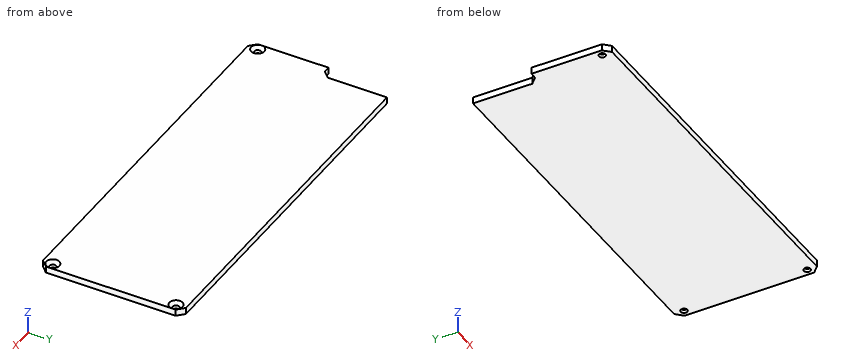
Autodesk Inventor part; units mm, degrees
ref_plane "YZ Plane" through (0, 0, 0) normal (1, 0, 0) x (0, 1, 0)
ref_plane "XZ Plane" through (0, 0, 0) normal (0, 1, 0) x (-1, 0, 0)
ref_plane "XY Plane" through (0, 0, 0) normal (0, 0, 1) x (1, 0, 0)
sketch "Sketch1" plane through (0, 0, 0) normal (1, 0, 0) x (0, 1, 0)
  point P0 (0, 0)
sketch "Sketch2" plane through (0, 0, 0) normal (0, 0, 1) x (1, 0, 0)
  line L0 (-65.94, 18.9) -> (48.46, 18.9)
  line L1 (48.46, 18.9) -> (48.46, -24.5)
  line L2 (48.46, -24.5) -> (-65.94, -24.5)
  line L3 (-65.94, -24.5) -> (-65.94, 18.9)
  point P0 (0, 0)
  dimension "d0" = 43.4
  dimension "d1" = 114.4
extrude "Extrusion1" add sketch "Sketch2" along normal blind 2
chamfer "Chamfer1" distance 2 angle 45 3 edges at (48.46, 18.9, 1) (48.46, -24.5, 1) (-65.94, -24.5, 1)
sketch "Sketch3" plane through (0, 0, 2) normal (0, 0, 1) x (1, 0, 0)
  line L0 (-65.94, 18.9) -> (-61.94, 18.9)
  line L1 (-61.94, 18.9) -> (-61.94, -1.1)
  line L2 (-61.94, -1.1) -> (-65.94, -1.1)
  line L3 (-65.94, -1.1) -> (-65.94, 18.9)
  point P0 (0, 0)
  dimension "d7" = 4
  dimension "d8" = 20
extrude "Extrusion2" cut sketch "Sketch3" against normal blind 2
chamfer "Chamfer2" distance 2 angle 45 1 edges at (-61.94, -1.1, 1)
sketch "Sketch4" plane through (0, 0, 2) normal (0, 0, 1) x (1, 0, 0)
  line L0 (-61.94, 18.9) -> (46.46, 18.9)
  line L1 (-63.94, -24.5) -> (46.46, -24.5)
  line L2 (48.46, -22.5) -> (48.46, 16.9)
  line L3 (-65.94, -22.5) -> (-65.94, -1.1)
  point P0 (0, 0)
  point P1 (-63.94, -21.5)
  point P2 (46.46, -21.5)
  point P3 (46.46, 15.9)
  dimension "d14" = 3
  dimension "d15" = 3
  dimension "d16" = 2
  dimension "d17" = 2
  dimension "d18" = 2
  dimension "d19" = 3
hole "Hole1" at (-63.94, -21.5, 2) at (46.46, -21.5, 2) at (46.46, 15.9, 2) direction (0, 0, -1) diameter 2 depth 8 tip angle 118 countersink diameter 4 countersink angle 90
properties part number "main body cover"
Source: CAD feature listing. Evaluate the final solid. Frame: model axes, mm. Round coordinates to 2 decimals unless told otherwise and drop trailing zeros. Write each loop counter-clockwise with the first axis right and the second up, starting at its lowest first coordinate (ties: lowest second). Pieces come first, ordered by that corner, then holes. Notation, with made-up numbers: M 23,62.25 L 81,62.25 A15 cw 81,77.25 Z; hole C 17.5,-22 d5. An arc over 180 degrees is marked long. Use CSV: the item, a comma, the result in double quotes. Start each with the question number.
Q1. Cut plane B-B on y = 6. Output: boundary loops of the cut face in (x, z), plus the area to 3 significant figures.
Q2. Line query: line 1 (X direction, y = -21.5, z = 0.5); line 2 (Y direction, x = 46.46, z = 0.2); line 3 (X direction, y = 15.9, z = 0.4). Output: solid intervals per line, ascending. Write a range as from..to.
Q3. Cut plane A-A on z = 1.4. Output: boundary loops of the cut face in (x, y).
Q4. First-contact query: P1, Ø2.5, axis at x = 46.46, y = 15.9, coming from the -Z side; P2, Ø3, axis at x = -63.94, y = -21.5, coming from the +Z side; P3, Ø1.6, axis at x = 46.46, y = -21.5, coming from the -Z side (1 decimal). Flat tips, straight axial feed; report the tip coordinate or a pass-through.
Results found:
1,outline,"M -61.94,0 L 48.46,0 L 48.46,2 L -61.94,2 Z"
1,area,"221 mm^2"
2,line 1,"-65.94..-64.94, -62.94..45.46, 47.46..48.46"
2,line 2,"-24.5..-22.5, -20.5..14.9, 16.9..18.9"
2,line 3,"-61.94..45.46, 47.46..48.46"
3,outline,"M -65.94,-22.5 L -63.94,-24.5 L 46.46,-24.5 L 48.46,-22.5 L 48.46,16.9 L 46.46,18.9 L -61.94,18.9 L -61.94,0.9 L -63.94,-1.1 L -65.94,-1.1 Z; hole C -63.94,-21.5 d2.8; hole C 46.46,-21.5 d2.8; hole C 46.46,15.9 d2.8"
4,P1,"z = 0"
4,P2,"z = 1.5"
4,P3,"through"
